```python
from build123d import *

# Parameters (mm, degrees)
PAD_DEPTH          = 30
POCKET_DEPTH       = 1167.961349
POLARPATTERN_COUNT = 3
CHAMFER_SIZE       = 10
FILLET_R           = 10


with BuildPart() as part:
    # Sketch → Pad (new body)
    with BuildSketch(Plane.XY):
        with BuildLine():
            Line((103.923048, -160), (190.525589, -10))
            ThreePointArc((190.525589, -10), (190.525589, 110), (86.60254, 170))
            Line((86.60254, 170), (-86.60254, 170))
            ThreePointArc((-86.60254, 170), (-190.525589, 110), (-190.525589, -10))
            Line((-190.525589, -10), (-103.923048, -160))
            ThreePointArc((-103.923048, -160), (0, -220), (103.923048, -160))
        make_face()
    extrude(amount=PAD_DEPTH)

    # Sketch001 (on Face8 of Pad) → Pocket (cut, through all)
    with BuildSketch(Plane.XY.offset(30)):
        with BuildLine():
            ThreePointArc((-40, -69.282032), (-67.320508, -76.60254), (-60, -103.923048))
            ThreePointArc((-60, -103.923048), (0, -120), (60, -103.923048))
            ThreePointArc((60, -103.923048), (67.320508, -76.60254), (40, -69.282032))
            ThreePointArc((-40, -69.282032), (0, -80), (40, -69.282032))
        make_face()
    pocket = extrude(amount=-POCKET_DEPTH, mode=Mode.SUBTRACT)

    # PolarPattern: Pocket ×3 about axis
    polarpattern_axis = Axis((0, 0, 30), (0, 0, 1))
    for i in range(1, POLARPATTERN_COUNT):
        add(pocket.rotate(polarpattern_axis, i * 360 / POLARPATTERN_COUNT), mode=Mode.SUBTRACT)

    # Chamfer
    chamfer_edges = [part.edges().sort_by_distance(p)[0] for p in [
        (69.282032, 40, 30),
        (0, -80, 30),
        (-69.282032, 40, 30),
    ]]
    chamfer(chamfer_edges, length=CHAMFER_SIZE)

    # Fillet
    fillet_edges = [part.edges().sort_by_distance(p)[0] for p in [
        (0, -220, 30),
    ]]
    fillet(fillet_edges, radius=FILLET_R)


solid = part.part
```
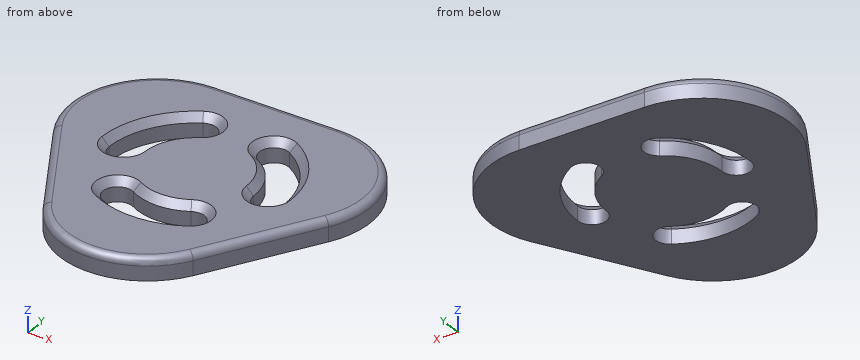
Build history of the part. All positions in model axes, mm. Give positions to 0.01 mm unless a question says otherwise; leave off trailing zeros. Loops run counter-clockwise (first coordinate to the right, second up) from the corner with the lowest first, then second, coordinate; pieces in that order, holes last. Notation, with made-up numbers: (47.5, 8.5) -> (94.5, 8.5) arc R10 ccw to (94.5, 22.5) -> close; hole circle Ø8 at (25.25, 51.25). An arc over 180 degrees is marked (long way). One line per question, with ' | ' between items.
Q1. Cut at A-A, the plane z = 12. Write the cut outline in (x, y), plus the area to 3 significant figures.
Filled sheet:
outline: (-190.53, -10) -> (-103.92, -160) arc R120 ccw to (103.92, -160) -> (190.53, -10) arc R120 ccw to (86.6, 170) -> (-86.6, 170) arc R120 ccw to start; hole (-120, 0) arc R20 ccw to (-80, 0) arc R80 cw to (-40, 69.28) arc R20 ccw to (-60, 103.92) arc R120 ccw to start; hole (-60, -103.92) arc R120 ccw to (60, -103.92) arc R20 ccw to (40, -69.28) arc R80 cw to (-40, -69.28) arc R20 ccw to start; hole (40, 69.28) arc R80 cw to (80, 0) arc R20 ccw to (120, 0) arc R120 ccw to (60, 103.92) arc R20 ccw to start | area: 104,000 mm²
Q2. Drop flat-ended pins along their axis: pin 1 (10 mm diameter, centred on y = -164.5, z = 11.5, fed in from +X); pin 2 (1 mm diameter, centred on x = -126.5, z = 10, fed in from +Y); pin 3 (10 mm diameter, centred on y = 99.5, z = 11.5, fed in from +X). Give the stop position or say it passes through.
Filled sheet:
pin 1: stops at x = 104.21 | pin 2: stops at y = 163.35 | pin 3: stops at x = 198.05
Q3. Drill centre lines: line 1 along Y through (x, z) = (58.5, 3); line 2 along Y through (x, z) = (-58, 12); line 3 along X through (y, z) = (2, 27.5). Where is each one in solid material? Low to high. Write a range as [from, to].
Filled sheet:
line 1: y = [-204.77, -104.77], [-68.5, 54.57], [104.71, 170] | line 2: y = [-205.05, -105.05], [-68.27, 55.1], [104.93, 170] | line 3: x = [-192.88, -127.48], [-72.47, 72.47], [127.48, 192.88]
Q4. Cut at B-B, the plane x = -50. Count the separate pieces of the cut face and the enclosed holes in it, plus the area to 3 significant figures.
Filled sheet:
separate pieces: 3 | enclosed holes: 0 | area: 8,510 mm²
